The model under review builds one solid part; all positions refer to its coordinate system, in mm. A direction names the side the tool comes from. Coordinates: 2 decimals unless noted, no trailing zeros. Loops run counter-clockwise (first coordinate to the right, second up) from the corner with the lowest first, then second, coordinate; pieces in that order, holes last. Notation, with made-up numbers: M -0.5,12.5 L 16.5,12.5 A15 cw 16.5,35.5 Z; hole C -7,-35.5 d7. An arc over 180 degrees is marked long. One line per item, written item: value.
Autodesk Inventor part; units mm, degrees
ref_plane "YZ Plane" through (0, 0, 0) normal (1, 0, 0) x (0, 1, 0)
ref_plane "XZ Plane" through (0, 0, 0) normal (0, 1, 0) x (-1, 0, 0)
ref_plane "XY Plane" through (0, 0, 0) normal (0, 0, 1) x (1, 0, 0)
sketch "Sketch1" plane through (0, 0, 0) normal (0, 1, 0) x (-1, 0, 0)
  line L0 (-26.5, 34) -> (26.5, 34)
  line L1 (26.5, 34) -> (26.5, -34)
  line L2 (26.5, -34) -> (-26.5, -34)
  line L3 (-26.5, -34) -> (-26.5, 34)
  line L4 (-26.5, 34) -> (26.5, -34) construction
  line L5 (26.5, 34) -> (-26.5, -34) construction
  line L6 (26.5, 34) -> (26.5, 19)
  line L7 (-26.5, -34) -> (-19.5, -34)
  line L8 (-26.5, -34) -> (8.5, -34)
  circle A0 centre (8.5, -31.5) radius 1.5
  circle A1 centre (-19.5, -31.5) radius 1.5
  line L9 (-19.5, -33) -> (-19.5, -34)
  line L10 (8.5, -33) -> (8.5, -34)
  circle A2 centre (-19.5, -31.5) radius 1.5
  circle A3 centre (24, 19) radius 1.5
  line L11 (25.5, 19) -> (26.5, 19)
  line L12 (26.5, 19) -> (25.5, 19)
  point P0 (0, 0)
  dimension "d6" = 3
  dimension "d7" = 3
  dimension "d9" = 3
  dimension "d0" = 53
  dimension "d1" = 68
  dimension "d2" = 15
  dimension "d3" = 7
  dimension "d4" = 35
  dimension "d12" = 1
  dimension "d13" = 1
sketch "Sketch2" plane through (0, 0, 0) normal (0, 1, 0) x (-1, 0, 0)
  line L0 (0, 0) -> (0, 34)
  line L1 (0, 34) -> (0, 21.5)
  line L2 (0, 21.5) -> (26.5, 21.5)
  line L3 (26.5, 21.5) -> (26.5, -34)
  line L4 (26.5, -34) -> (-22, -34)
  line L5 (-22, -34) -> (-22, 21.5)
  line L6 (-22, 21.5) -> (0, 21.5)
  line L7 (26.5, 21.5) -> (26.5, 16.5)
  line L8 (21.5, 16.5) -> (-22, 16.5)
  line L9 (-22, 16.5) -> (-17, 16.5)
  line L10 (-22, 21.5) -> (-17, 21.5)
  line L11 (-17, 16.5) -> (-17, -29)
  line L12 (-22, -34) -> (-22, -29)
  line L13 (-17, -29) -> (21.5, -29)
  line L14 (26.5, -34) -> (21.5, -34)
  line L15 (21.5, -29) -> (21.5, 16.5)
  circle A0 centre (24, 19) radius 1.5
  line L16 (21.5, -29) -> (8.5, -29)
  line L17 (8.5, -29) -> (8.5, -31.5)
  circle A1 centre (8.5, -31.5) radius 1.5
  circle A2 centre (-19.5, -31.5) radius 1.5
  circle A3 centre (8.5, -31.5) radius 1.5
  line L18 (26.5, 21.5) -> (25.0607, 20.0607)
  line L19 (-17, -29) -> (-18.4393, -30.4393)
  line L20 (-20.5607, -32.5607) -> (-22, -34)
  point P0 (-17, -6.25)
  dimension "d25" = 3
  dimension "d14" = 34
  dimension "d15" = 12.5
  dimension "d16" = 26.5
  dimension "d17" = 55.5
  dimension "d18" = 48.5
  dimension "d19" = 55.5
  dimension "d20" = 5
  dimension "d21" = 48.5
  dimension "d23" = 5
  dimension "d24" = 5
  dimension "d26" = 13
  dimension "d27" = 3
  dimension "d28" = 3
  dimension "d29" = 3
extrude "Extrusion1" add sketch "Sketch2" along normal blind 4 contours L8 L5 L6 L0 | L0 L2 L3 L4 L20 A2 L19 L13 L15 L8 | L11 L19 A2 L20 L5 L8
extrude "Extrusion2" add sketch "Sketch1" against normal blind 3
properties part number "Arduino_Screw_Hole_Base"
(1) Add section B-B on x = 19.5. State the section outline as (y, z) points.
Checks:
outline: M -3,-34 L 4,-34 L 4,-33 L -3,-33 Z; M -3,-30 L 4,-30 L 4,21.5 L 0,21.5 L 0,34 L -3,34 Z
(2) Add section A-A on z = -31.5. State the section outline as (x, y) points, then the cut area to 3 significant figures.
Checks:
outline: M -26.5,-3 L -10,-3 L -10,4 L -26.5,4 Z; M -7,-3 L 18,-3 L 18,4 L -7,4 Z; M 21,-3 L 26.5,-3 L 26.5,0 L 22,0 L 22,4 L 21,4 Z
area: 311 mm^2
(3) Tool access review of faces 4 (the face through (17, 2, -6)), 5 (the face through (-7.39, 0.55, -30.49)), 6 (the face through (-2, 2, 21.5)): name each direction out of +Z, -Z, +X, -X, +Y, -Y from which nothing blocks a thin tool from reaching the whole face with its end or side.
Checks:
face 4: +Y
face 5: +Y, -Y
face 6: +Z, +X, -X, +Y
(4) Add section D-D on x = -8.5. State the section outline as (y, z) points, then the cut area to 3 significant figures.
Checks:
outline: M -3,-34 L 4,-34 L 4,-33 L -3,-33 Z; M -3,-30 L 4,-30 L 4,-29 L 0,-29 L 0,16.5 L 4,16.5 L 4,21.5 L 0,21.5 L 0,34 L -3,34 Z
area: 223 mm^2
(5) To check wall thickness, follow L1, parallel to X at y = 0.25, z = -3.5; L2, parallel to Z at x = -24, y = 1.75; L3, parallel to Z at x = -8.5, y = -1.5. State the ranges of each line that lie inside material, in increasing order. Write a range as [from, to].
Checks:
L1: [-26.5, -21.5], [17, 22]
L2: [-34, 17.5], [20.5, 21.5]
L3: [-34, -33], [-30, 34]
(6) Insertion check: pin 1 Ø11.5 at (x, z) = (-0.5, -16) entering from +Y; pin 2 Ø3 at (y, z) = (2, 4) entering from +X; pin 3 Ø1.2 at (x, y) = (3, 2.5) entering from +Z. Each pin has a flat end and moves straight along its axis. Give the tip position at first contact, or say it passes through.
Checks:
pin 1: y = 0
pin 2: x = 22
pin 3: z = 21.5
(7) Add section C-C on y = 3.25. State the section outline as (x, z) points.
Checks:
outline: M -26.5,-34 L 22,-34 L 22,21.5 L -26.5,21.5 Z; hole C -24,19 d3; hole M -21.5,-29 L 17,-29 L 17,16.5 L -21.5,16.5 Z; hole C -8.5,-31.5 d3; hole C 19.5,-31.5 d3
(8) Draft analysis for pull direction X (two halves, no side actions). For faces 1 (the face through (-3, 2, 16.5)), 2 (the face through (0, -1, 34)), 3 (the face through (22, 2, -7)), state which applies: pulls with the +X half, pulls with the -X half, needs draft (parallel to the pull), parting line crosses it, or undercut.
Checks:
face 1: undercut
face 2: needs draft
face 3: pulls with the +X half
